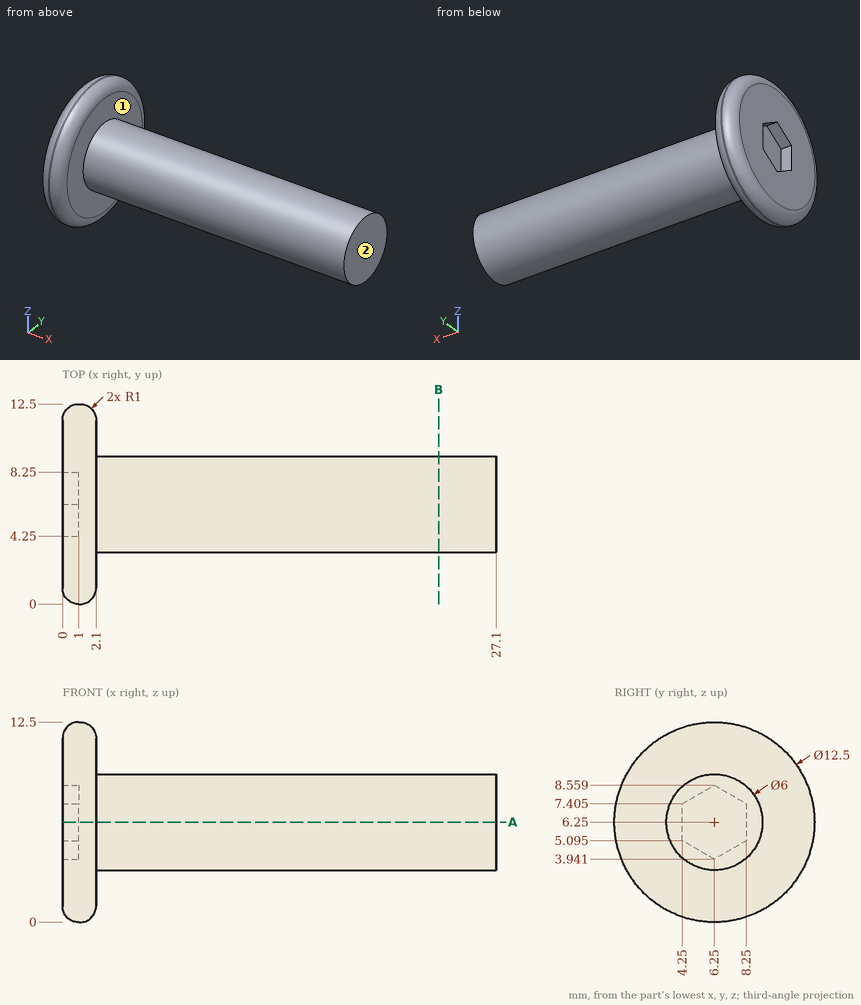
Here's the drawing with two shaded views (mm, measured from the low corner). I have some questions. A direction names the side the tool comes from. Give positions to 0.01 mm unless a question says otherwise; leave off trailing zeros. Order: outer loops, then holes, each group sorted by start corner. A loop starts at its lowest first (then second) coordinate and runs counter-clockwise, first axis right, second up. Notation, with made-up numbers: (-37, 13) - (-6, 13) arc R13 cw to (-6, 25) - close; hole circle Ø5 at (10.25, -4.5). An arc over 180 degrees is marked (long way). Write each question's results on one line, items separated by ' | '.
1) I'm going to push flat-ended pins straight in: pin 1 Ø5 at (x, z) = (13.5, 5.5) entering from +Y; pin 2 Ø1 at (y, z) = (5, 7) entering from -X; pin 3 Ø6 at (x, z) = (24, 2) entering from -Y; pin 4 Ø3 at (y, z) = (6, 2) entering from -X. Where does each tip first touch, or does it pass through?
Final values:
pin 1: stops at y = 9.25 | pin 2: stops at x = 1 | pin 3: stops at y = 3.52 | pin 4: stops at x = 0
2) Suppose I cut it at A-A, the plane z = 6.25. Write out the boundary of the cut face in (x, y), then the cut area to 3 significant figures.
Final values:
outline: (0, 1) arc R1 ccw to (1, 0) - (1.1, 0) arc R1 ccw to (2.1, 1) - (2.1, 3.25) - (27.1, 3.25) - (27.1, 9.25) - (2.1, 9.25) - (2.1, 11.5) arc R1 ccw to (1.1, 12.5) - (1, 12.5) arc R1 ccw to (0, 11.5) - (0, 8.25) - (1, 8.25) - (1, 4.25) - (0, 4.25) - close | area: 171 mm^2
3) On a 3-axis mill with a long thin cutter (end or side, diameter ignored), from which of +Z, -Z, +X, -X, +Y, -Y can I reach the whole of each face in a straight line? I mean the marked faces 1 and 2. Say none if no direction works.
Final values:
face 1: +X | face 2: +Z, -Z, +X, +Y, -Y
4) Suppose I cut it at B-B, the plane x = 23.5. Write out the boundary of the cut face in (y, z).
Final values:
outline: circle Ø6 at (6.25, 6.25)
5) Please list where these lines run through material, in increasing order: line 1 along X through (y, z) = (10, 5.5); line 2 along Y through (x, z) = (23, 7.5); line 3 along Y through (x, z) = (23.25, 4.75). Write a range as [from, to].
Final values:
line 1: x = [0, 2.1] | line 2: y = [3.52, 8.98] | line 3: y = [3.65, 8.85]
